Geometry: final body of the model. Coordinates: model frame, mm. Face numbers are marked on the shaded views. Give positions to 0.01 mm unless a question says otherwise; leave off trailing zeros. Write each loop counter-clockwise with the first axis right and the second up, starting at its lowest first coordinate (ties: lowest second). Pieces come first, ordered by that corner, then holes.
from build123d import *

# Parameters (mm, degrees)
SKETCH1_W                      = 22
SKETCH1_H                      = 18
BOSS_EXTRUDE1_DEPTH            = 3
CUT_EXTRUDE1_REACH             = 5
SKETCH2_R                      = 1.75
CUT_EXTRUDE1_DIRECTION_2_DEPTH = 1
CHAMFER1_SIZE                  = 2


with BuildPart() as part:
    # Sketch1 → Boss-Extrude1 (new body)
    with BuildSketch(Plane(origin=(0, 0, 0), x_dir=(1, 0, 0), z_dir=(0, 1, 0))):
        Rectangle(SKETCH1_W, SKETCH1_H)
    extrude(amount=BOSS_EXTRUDE1_DEPTH)

    # Sketch2 → Cut-Extrude1 (cut, up to next)
    with BuildSketch(Plane(origin=(0, 3, 0), x_dir=(1, 0, 0), z_dir=(0, 1, 0)), mode=Mode.PRIVATE) as cut_extrude1_sk1:
        with Locations((0, 6)):
            Circle(SKETCH2_R)
    cut_extrude1_tool1 = extrude(cut_extrude1_sk1.sketch, amount=-CUT_EXTRUDE1_REACH, mode=Mode.PRIVATE) & part.part
    add(cut_extrude1_tool1.solids().sort_by_distance((0, 3, -6))[0], mode=Mode.SUBTRACT)
    # Sketch2 → Cut-Extrude1 (cut, up to next)
    with BuildSketch(Plane(origin=(0, 3, 0), x_dir=(1, 0, 0), z_dir=(0, 1, 0)), mode=Mode.PRIVATE) as cut_extrude1_sk2:
        with Locations((0, -6)):
            Circle(SKETCH2_R)
    cut_extrude1_tool2 = extrude(cut_extrude1_sk2.sketch, amount=-CUT_EXTRUDE1_REACH, mode=Mode.PRIVATE) & part.part
    add(cut_extrude1_tool2.solids().sort_by_distance((0, 3, 6))[0], mode=Mode.SUBTRACT)

    # Sketch2 → Cut-Extrude1 direction 2 (cut)
    with BuildSketch(Plane(origin=(0, 3, 0), x_dir=(1, 0, 0), z_dir=(0, 1, 0))):
        with Locations((0, 6)):
            Circle(SKETCH2_R)
        with Locations((0, -6)):
            Circle(SKETCH2_R)
    extrude(amount=CUT_EXTRUDE1_DIRECTION_2_DEPTH, mode=Mode.SUBTRACT)

    # Chamfer1
    chamfer1_edges = [part.edges().sort_by_distance(p)[0] for p in [
        (11, 1.5, 9),
        (-11, 1.5, 9),
        (-11, 1.5, -9),
        (11, 1.5, -9),
    ]]
    chamfer(chamfer1_edges, length=CHAMFER1_SIZE)


solid = part.part
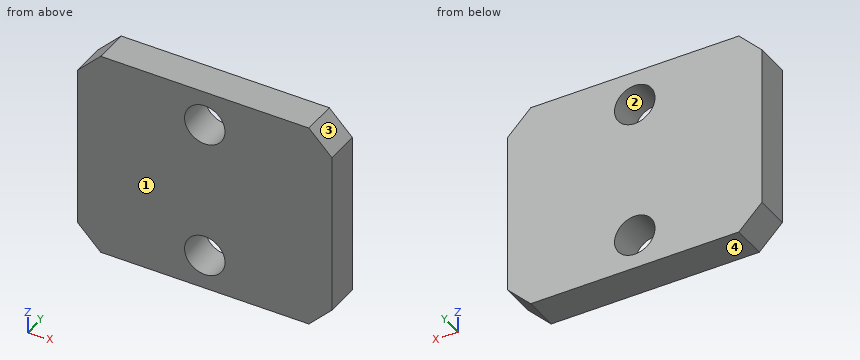
Q1. Section C-C on y = 1.2. Output: boundary loops of the cut face in (x, z), plus the area to 3 significant figures.
Filled sheet:
outline: (-11, -7) - (-9, -9) - (9, -9) - (11, -7) - (11, 7) - (9, 9) - (-9, 9) - (-11, 7) - close; hole circle Ø3.5 at (0, -6); hole circle Ø3.5 at (0, 6)
area: 369 mm2
Q2. Section A-A on x = 0. Output: boundary loops of the cut face in (y, z), plus the area to 3 significant figures.
Filled sheet:
outline: (0, -9) - (3, -9) - (3, -7.75) - (0, -7.75) - close; (0, -4.25) - (3, -4.25) - (3, 4.25) - (0, 4.25) - close; (0, 7.75) - (3, 7.75) - (3, 9) - (0, 9) - close
area: 33.0 mm2
Q3. Section B-B on z = -6. Output: boundary loops of the cut face in (x, y), plus the area to 3 significant figures.
Filled sheet:
outline: (-11, 0) - (-1.75, 0) - (-1.75, 3) - (-11, 3) - close; (1.75, 0) - (11, 0) - (11, 3) - (1.75, 3) - close
area: 55.5 mm2
Q4. Ray query, line 1 along Z through (x, y) = (0, 0.8); line 2 along X through (y, z) = (0.75, 6); line 3 along Z through (x, y) = (-1.5, 0.55). Return the intervals inside material, ascending.
Filled sheet:
line 1: z = -9 to -7.75, -4.25 to 4.25, 7.75 to 9
line 2: x = -11 to -1.75, 1.75 to 11
line 3: z = -9 to -6.9, -5.1 to 5.1, 6.9 to 9
Q5. Pull-direction query (Z, two-part tool) for the marked faces 1, 2, 3 and 4; classes: released by +Z, released by -Z, zero draft, split by the parting line, or undercut.
Filled sheet:
face 1: zero draft
face 2: undercut
face 3: released by +Z
face 4: released by -Z
Q6. Section D-D on x = -9.25. Output: boundary loops of the cut face in (y, z).
Filled sheet:
outline: (0, -8.75) - (3, -8.75) - (3, 8.75) - (0, 8.75) - close
Q7. Pin query (flat end, axial travel): P1, Ø3, axis at x = 0, z = -6, coming from the +Y side. Return the tip coordinate at first contact, or that it passes through.
Filled sheet:
P1: passes through
